Autodesk Inventor part; units mm, degrees
ref_plane "YZ Plane" through (0, 0, 0) normal (1, 0, 0) x (0, 1, 0)
ref_plane "XZ Plane" through (0, 0, 0) normal (0, 1, 0) x (-1, 0, 0)
ref_plane "XY Plane" through (0, 0, 0) normal (0, 0, 1) x (1, 0, 0)
sketch "Sketch1" plane through (0, 0, 0) normal (0, 0, 1) x (1, 0, 0)
  circle A0 centre (0, 0) radius 25.4
  dimension "d0" = 50.8
extrude "Extrusion1" add sketch "Sketch1" along normal mid plane 381
sketch "Sketch4" plane through (0, 0, 190.5) normal (0, 0, 1) x (1, 0, 0)
  line L0 (-12.7, 20.6375) -> (12.7, 20.6375)
  line L1 (12.7, 20.6375) -> (12.7, -20.6375)
  line L2 (12.7, -20.6375) -> (-12.7, -20.6375)
  line L3 (-12.7, -20.6375) -> (-12.7, 20.6375)
  line L4 (-12.7, 20.6375) -> (12.7, -20.6375) construction
  line L5 (12.7, 20.6375) -> (-12.7, -20.6375) construction
  point P0 (0, 0)
  dimension "d15" = 25.4
  dimension "d16" = 41.275
extrude "Extrusion4" add sketch "Sketch4" along normal blind 50.8
fillet "Fillet2" radius 20.6375 2 edges at (0, 20.6375, 241.3) (0, -20.6375, 241.3)
sketch "Sketch5" plane through (12.7, -20.6375, 190.5) normal (1, 0, 0) x (0, 0, -1)
  arc A0 (-30.1625, 41.275) -> (-30.1625, 0) centre (-30.1625, 20.6375) ccw
  circle A1 centre (-30.1625, 20.6375) radius 9.525
  point P0 (190.5, 20.6375)
extrude "Extrusion5" cut sketch "Sketch5" against normal blind 50.8
mirror "Mirror1" about plane through (0, 0, 0) normal (0, 0, 1) of "Extrusion4", "Fillet2", "Extrusion5"
properties part number "body to wheel hub connectors (19 in)"
Design review of the part built by this model. Coordinates are the model's own, in mm. A direction names the side the tool comes from. Give positions to 0.01 mm unless a question says otherwise; leave off trailing zeros. Write each loop counter-clockwise with the first axis right and the second up, starting at its lowest first coordinate (ties: lowest second). Pieces come first, ordered by that corner, then holes. Notation, with made-up numbers: M -4.5,84.25 L 23.5,84.25 A13 cw 23.5,98.25 Z; hole C 72,49 d3. An arc over 180 degrees is marked long. Return JSON: item names as keys, results as strings. Group by question number.
Item 1: Take a section at B-B (z = 15). Give the boundary of the cut face in (x, y).
Item 2: Take a section at A-A (x = 0). Count the separate pieces of the cut face and the enclosed holes in it, plus the area to 3 significant figures.
Item 3: The part is to be moulded in two halves that separate along Z. For faces 6 (the cylindrical face through (0.178, -3.648, 211.864)), 7 (the cylindrical face through (0.178, 3.648, -211.864)), 8 (the flat face through (12.7, 0, 210)), 9 (the cylindrical face through (0.178, 14.753, 235.094)), say which applies: pulls with the +Z half, pulls with the -Z half, needs draft (parallel to the pull), parting line crosses it, or undercut.
Item 4: Take a section at D-D (z = 200). Give the boundary of the cut face in (x, y), plus the area to 3 significant figures.
Item 5: Take a section at C-C (x = -20.5). Give the boundary of the cut face in (y, z), plus the area to 3 significant figures.
Item 6: Clearance check with flat-ended pins moving along their axes: pin 1 Ø20.5 at (y, z) = (0, 208.5) entering from -X; pin 2 Ø6 at (y, z) = (8.5, -77) entering from -X; pin 3 Ø20.5 at (x, z) = (-4.5, 201) entering from +Y; pin 4 Ø17 at (y, z) = (0, -220.66) entering from +X. State where each tip first meets the part, or that it passes through.
Item 7: Wall thickness on line 1 along Z through (x, y) = (-4.5, 0.5); line 2 along X through (y, z) = (2, 203); line 3 along Z through (x, y) = (-16.5, -1): over which ranges is each line inside the solid? List them lowest first.
Item 8: Tool access review of faces 1 (the flat face through (0, -20.638, 205)), 2 (the flat face through (0, 20.638, 205)), 3 (the flat face through (-12.7, 0, -210)), 4 (the flat face through (0, -20.638, -205)), 5 (the flat face through (0, 20.638, -205)): name each direction out of +Z, -Z, +X, -X, +Y, -Y from which nothing blocks a thin tool from reaching the whole face with its end or side.
Return value:
{
 "1": {"outline": "C 0,0 d50.8"},
 "2": {"separate pieces": "1", "enclosed holes": "2", "area": "22,600 mm2"},
 "3": {"face 6": "undercut", "face 7": "undercut", "face 8": "needs draft", "face 9": "pulls with the +Z half"},
 "4": {"outline": "M -12.7,-20.64 L 12.7,-20.64 L 12.7,20.64 L -12.7,20.64 Z", "area": "1,050 mm2"},
 "5": {"outline": "M -15,-190.5 L 15,-190.5 L 15,190.5 L -15,190.5 Z", "area": "11,400 mm2"},
 "6": {"pin 1": "stops at x = -12.7", "pin 2": "stops at x = -24.8", "pin 3": "stops at y = 20.64", "pin 4": "passes through"},
 "7": {"line 1": "z = -241.29 to -230.17, -211.15 to 211.15, 230.17 to 241.29", "line 2": "x = -12.7 to 12.7", "line 3": "z = -190.5 to 190.5"},
 "8": {"face 1": "+Z, +X, -X, -Y", "face 2": "+Z, +X, -X, +Y", "face 3": "-Z, -X, +Y, -Y", "face 4": "-Z, +X, -X, -Y", "face 5": "-Z, +X, -X, +Y"}
}
